The listing builds one solid part. Answer for the finished solid, in the listing's coordinates (mm). A direction names the side the tool comes from. Give positions to 0.01 mm unless a question says otherwise; leave off trailing zeros. Order: outer loops, then holes, each group sorted by start corner. A loop starts at its lowest first (then second) coordinate and runs counter-clockwise, first axis right, second up. Notation, with made-up numbers: (73.25, -35.5) - (123.25, -35.5) arc R6 cw to (123.25, -31.5) - close; hole circle Ø2 at (56, -11.75). An arc over 180 degrees is marked (long way). Answer as a JSON object with one key per item and string values. Group by question number.
Q1. Consider line 1 (Z direction, x = -15.25, y = 24); line 2 (X direction, y = 244, z = 9); line 3 (Z direction, x = -1, y = 161.5). Determine where each line is inside the solid, lowest interval first.
Q2. For faces 4 (the face through (0.805, 12.673, 8.351)), 5 (the face through (0, 182, 10)), determine the directions among +Z, -Z, +X, -X, +Y, -Y from which every point of the face is accessible in a straight line to the end or side of a thin tool.
Q3. Given pin 1 (10 mm diameter, centred on x = -2.5, z = 11, fed in from +Y); pin 2 (3 mm diameter, centred on y = 74.5, z = 8.5, fed in from -X); pin 3 (5.5 mm diameter, centred on x = -7.94, y = 9.52, fed in from +Z), each flat-ended and moving along its own axis, determine where each tip first touches the part or whether it passes through.
Q4. A cutting plane is placed at A-A, the plane z = 7.75. Give the vertices of the cut face in (x, y), and give its area (3 significant figures).
Q5. A cutting plane is placed at B-B, the plane y = 62. Give the vertices of the cut face in (x, z) (1 decimal), and give its area (3 significant figures).
Q6. The mould has two halves that part along Y. Classify faces 1 (the face through (-3.7, 0, -0.5)), 2 (the face through (-9.644, 12.202, -0.805)), 3 (the face through (-8, 182, -1.588)): released by +Y, released by -Y, zero draft, split by the parting line, or undercut.
Autodesk Inventor part; units mm, degrees
ref_plane "YZ Plane" through (0, 0, 0) normal (1, 0, 0) x (0, 1, 0)
ref_plane "XZ Plane" through (0, 0, 0) normal (0, 1, 0) x (-1, 0, 0)
ref_plane "XY Plane" through (0, 0, 0) normal (0, 0, 1) x (1, 0, 0)
sketch "Sketch1" plane through (0, 0, 0) normal (0, 1, 0) x (-1, 0, 0)
  line L0 (0, 17.4625) -> (0, 1.5875)
  line L1 (1.5875, 0) -> (17.4625, 0)
  line L2 (17.4625, 0) -> (17.4625, -1.5875)
  line L3 (17.4625, -1.5875) -> (-1.5875, -1.5875)
  line L4 (-1.5875, -1.5875) -> (-1.5875, 17.4625)
  line L5 (-1.5875, 17.4625) -> (0, 17.4625)
  arc A0 (0, 1.5875) -> (1.5875, 0) centre (1.5875, 1.5875) ccw
  point P0 (0, 0)
  dimension "d0" = 1.5875
  dimension "d1" = 19.05
  dimension "d2" = 1.5875
extrude "Extrusion1" add sketch "Sketch1" along normal blind 368.3
sketch "Sketch2" plane through (1.5875, 0, -1.5875) normal (0, 0, -1) x (-1, 0, 0)
  line L0 (19.05, 0) -> (0, 0) construction
  line L1 (9.525, 0) -> (9.525, 443.5725) construction
  circle A0 centre (9.525, 9.525) radius 3.175
  point P0 (1.5875, 0)
  dimension "d5" = 6.35
  dimension "d6" = 9.525
extrude "Extrusion2" cut sketch "Sketch2" against normal through all
sketch "Sketch3" plane through (1.5875, 0, 17.4625) normal (1, 0, 0) x (0, 0, -1)
  line L0 (19.05, 0) -> (0, 0) construction
  line L1 (9.525, 0) -> (9.525, 23.4407) construction
  circle A0 centre (9.525, 9.525) radius 3.175
  point P0 (17.4625, 0)
  dimension "d9" = 6.35
  dimension "d10" = 9.525
extrude "Extrusion3" cut sketch "Sketch3" against normal through all
properties part number "Long Wall Support" material "Aluminum 6061"
Reply:
{
 "1": {"line 1": "z = -1.59 to 0", "line 2": "x = 0 to 1.59", "line 3": "z = -1.59 to 0.11"},
 "2": {"face 4": "+X, -X", "face 5": "+Z, -X, +Y, -Y"},
 "3": {"pin 1": "stops at y = 368.3", "pin 2": "stops at x = 0", "pin 3": "passes through"},
 "4": {"outline": "(0, 0) - (1.59, 0) - (1.59, 6.36) - (0, 6.36) - close; (0, 12.69) - (1.59, 12.69) - (1.59, 368.3) - (0, 368.3) - close", "area": "575 mm^2"},
 "5": {"outline": "(-17.5, -1.6) - (1.6, -1.6) - (1.6, 17.5) - (0, 17.5) - (0, 1.6) arc R1.6 cw to (-1.6, 0) - (-17.5, 0) - close", "area": "58.5 mm^2"},
 "6": {"face 1": "released by -Y", "face 2": "undercut", "face 3": "zero draft"}
}
